Geometry check sheet. Reference: the model listing, model coordinates, mm. Coordinates: 2 decimals unless noted, no trailing zeros. Loops run counter-clockwise (first coordinate to the right, second up) from the corner with the lowest first, then second, coordinate; pieces in that order, holes last. Notation, with made-up numbers: (28.5, 54) - (33.5, 54) arc R26 cw to (33.5, 91) - close; hole circle Ø5 at (58, 9). An arc over 180 degrees is marked (long way). Write each question's results on one line, items separated by ' | '. Start each with the question number.
(1) Sectioned sample at A-A (z = 428). Enter the section's corners in (x, y).
(2) Sectioned sample at B-B (y = 26.5). Enter the section's corners in (x, z).
(3) Material ranges on probe 1 along Z at (x, y) = (-14, 1); probe 2 along X at (y, z) = (34.5, 116); probe 3 along X at (y, z) = (-6, 365.5), recorded low to high.
(4) Sectioned sample at C-C (x = -23.5). Enter the section's corners in (y, z), plus the area to 3 significant figures.
from build123d import *

# Parameters (mm, degrees)
F0_W        = 165.1
F0_H        = 800.1
F0_W_2      = 139.7
F0_H_2      = 596.9
F0_W_3      = 127
F0_H_3      = 571.5
F0_W_4      = 101.6
F0_H_4      = 546.1
F1_DEPTH    = 50.8
F2_DEPTH    = 5
F3_DEPTH    = 38.1
F4_R        = 50.79999
F2_FACE_W   = 165.1
F2_FACE_H   = 800.1
F2_FACE_W_2 = 139.7
F2_FACE_H_2 = 596.9
F5_DEPTH    = 10


# Not quite as in the source:
# - a fillet or chamfer is up to 0.001 mm smaller than in the source, because OpenCascade refuses the exact size
# - a feature names something its author has since deleted; it is built from what else it names


with BuildPart() as f1:
    # F0 (on Front) → F1 (new body)
    with BuildSketch(Plane.XZ):
        with Locations((0, 209.55)):
            Rectangle(F0_W, F0_H)
        with Locations((0, 298.45)):
            Rectangle(F0_W_2, F0_H_2, mode=Mode.SUBTRACT)
        with Locations((0, 298.45)):
            Rectangle(F0_W_2, F0_H_2)
        with Locations((0, 298.45)):
            Rectangle(F0_W_3, F0_H_3, mode=Mode.SUBTRACT)
        with Locations((0, 298.45)):
            Rectangle(F0_W_3, F0_H_3)
        with Locations((2.54, 298.45)):
            Rectangle(F0_W_4, F0_H_4, mode=Mode.SUBTRACT)
    extrude(amount=-F1_DEPTH)

    # F0 (on Front) → F2 (cut)
    with BuildSketch(Plane.XZ):
        with Locations((0, 298.45)):
            Rectangle(F0_W_2, F0_H_2)
        with Locations((0, 298.45)):
            Rectangle(F0_W_3, F0_H_3, mode=Mode.SUBTRACT)
    extrude(amount=-F2_DEPTH, mode=Mode.SUBTRACT)

    # F0 (on Front) → F3 (cut)
    with BuildSketch(Plane.XZ):
        with Locations((0, 298.45)):
            Rectangle(F0_W_3, F0_H_3)
        with Locations((2.54, 298.45)):
            Rectangle(F0_W_4, F0_H_4, mode=Mode.SUBTRACT)
    extrude(amount=-F3_DEPTH, mode=Mode.SUBTRACT)

    # F4 (radius 50.8 in the source; OpenCascade refuses exactly that, so slightly less here)
    f4_edges = [f1.edges().sort_by_distance(p)[0] for p in [
        (53.34, 44.45, 571.5),
        (-48.26, 44.45, 571.5),
        (-48.26, 44.45, 25.4),
        (53.34, 44.45, 25.4),
    ]]
    fillet(f4_edges, radius=F4_R)

    # F0 (on Front) + F2_face (on face) → F5 (join)
    with BuildSketch(Plane.XZ):
        with Locations((0, 209.55)):
            Rectangle(F0_W, F0_H)
        with Locations((0, 298.45)):
            Rectangle(F0_W_2, F0_H_2, mode=Mode.SUBTRACT)
    with BuildSketch(Plane(origin=(0, 0, 57.3602649007), x_dir=(1, 0, 0), z_dir=(0, -1, 0))):
        with Locations((0, 152.1897350993)):
            Rectangle(F2_FACE_W, F2_FACE_H)
        with Locations((0, 241.0897350993)):
            Rectangle(F2_FACE_W_2, F2_FACE_H_2, mode=Mode.SUBTRACT)
    extrude(amount=F5_DEPTH)


solid = f1.part
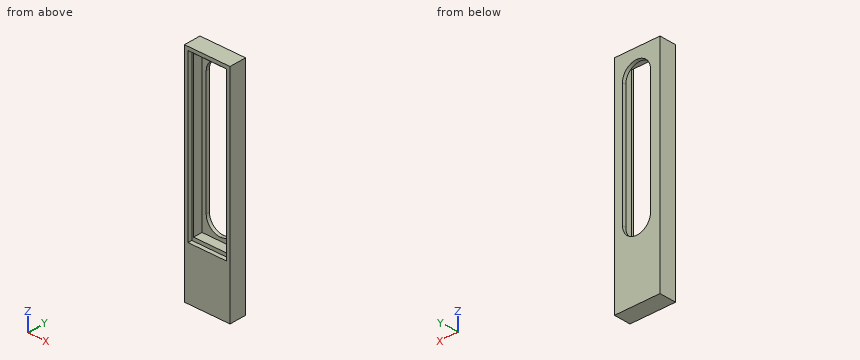
Outcome:
1) outline: (-82.55, -10) - (-69.85, -10) - (-69.85, 5) - (-63.5, 5) - (-63.5, 38.1) - (-48.26, 38.1) - (-48.26, 50.8) - (-82.55, 50.8) - close; (53.34, 38.1) - (63.5, 38.1) - (63.5, 5) - (69.85, 5) - (69.85, -10) - (82.55, -10) - (82.55, 50.8) - (53.34, 50.8) - close
2) outline: (-82.55, -190.5) - (82.55, -190.5) - (82.55, 609.6) - (-82.55, 609.6) - close; hole (-63.5, 12.7) - (63.5, 12.7) - (63.5, 584.2) - (-63.5, 584.2) - close
3) probe 1: z = -190.5 to 0, 596.9 to 609.6 | probe 2: x = -82.55 to -63.5, 63.5 to 82.55 | probe 3: x = -82.55 to -69.85, 69.85 to 82.55
4) outline: (-10, -190.5) - (50.8, -190.5) - (50.8, 32.58) - (38.1, 32.58) - (38.1, 12.7) - (5, 12.7) - (5, 0) - (-10, 0) - close; (-10, 596.9) - (5, 596.9) - (5, 584.2) - (38.1, 584.2) - (38.1, 564.32) - (50.8, 564.32) - (50.8, 609.6) - (-10, 609.6) - close | area: 14,000 mm2
